```python
from build123d import *

# Parameters (mm, degrees)
SKETCH_1_R          = 16
SKETCH_1_R_2        = 1.2
EXTRUDE_1_DEPTH     = 3.6
SKETCH_2_R          = 2
CUT_EXTRUDE_1_DEPTH = 2
SKETCH_3_R          = 1
CUT_EXTRUDE_2_DEPTH = 2
SKETCH_4_R          = 7.9
EXTRUDE_2_DEPTH     = 10
SKETCH_6_R          = 0.7
CUT_EXTRUDE_3_DEPTH = 5


with BuildPart() as part:
    # 스케치1 → 보스-돌출1 (new body)
    with BuildSketch(Plane.XY):
        Circle(SKETCH_1_R)
        with Locations((13, 0)):
            Circle(SKETCH_1_R_2, mode=Mode.SUBTRACT)
        with Locations((6.5, -11.258330249)):
            Circle(SKETCH_1_R_2, mode=Mode.SUBTRACT)
        with Locations((-6.5, -11.258330249)):
            Circle(SKETCH_1_R_2, mode=Mode.SUBTRACT)
        with Locations((-13, 0)):
            Circle(SKETCH_1_R_2, mode=Mode.SUBTRACT)
        with Locations((-6.5, 11.258330249)):
            Circle(SKETCH_1_R_2, mode=Mode.SUBTRACT)
        with Locations((6.5, 11.258330249)):
            Circle(SKETCH_1_R_2, mode=Mode.SUBTRACT)
    extrude(amount=EXTRUDE_1_DEPTH)

    # 스케치2 → 컷-돌출1 (cut)
    with BuildSketch(Plane.XY.offset(3.6)):
        with Locations((13, 0)):
            Circle(SKETCH_2_R)
        with Locations((6.5, -11.258330249)):
            Circle(SKETCH_2_R)
        with Locations((-6.5, -11.258330249)):
            Circle(SKETCH_2_R)
        with Locations((-13, 0)):
            Circle(SKETCH_2_R)
        with Locations((-6.5, 11.258330249)):
            Circle(SKETCH_2_R)
        with Locations((6.5, 11.258330249)):
            Circle(SKETCH_2_R)
    extrude(amount=-CUT_EXTRUDE_1_DEPTH, mode=Mode.SUBTRACT)

    # 스케치3 → 컷-돌출2 (cut)
    with BuildSketch(Plane(origin=(0, 0, 0), x_dir=(-1, 0, 0), z_dir=(0, 0, -1))):
        with Locations((-6, 0)):
            Circle(SKETCH_3_R)
        with Locations((6, 0)):
            Circle(SKETCH_3_R)
    extrude(amount=-CUT_EXTRUDE_2_DEPTH, mode=Mode.SUBTRACT)

    # 스케치4 → 보스-돌출2 (add)
    with BuildSketch(Plane.XY.offset(3.6)):
        Circle(SKETCH_4_R)
    extrude(amount=EXTRUDE_2_DEPTH)

    # 스케치5 → 컷-회전1 (revolve, cut)
    with BuildSketch(Plane(origin=(0, 0, 0), x_dir=(0, 0, -1), z_dir=(1, 0, 0))):
        Polygon((-13.6, 7.9), (-13.6, 5.9), (-12.35, 4.6), (-11.1, 5.9), (-11.1, 7.9), align=None)
        Polygon((-6.1, 7.9), (-3.6, 7.9), (-3.6, 5.9), (-4.85, 4.6), (-6.1, 5.9), align=None)
    revolve(axis=Axis((0, 0, 0), (0, 0, 1)), mode=Mode.SUBTRACT)

    # 스케치6 → 컷-돌출3 (cut)
    with BuildSketch(Plane.XY.offset(11.1)):
        with Locations((6.6, 0)):
            Circle(SKETCH_6_R)
    extrude(amount=-CUT_EXTRUDE_3_DEPTH, mode=Mode.SUBTRACT)


solid = part.part
```
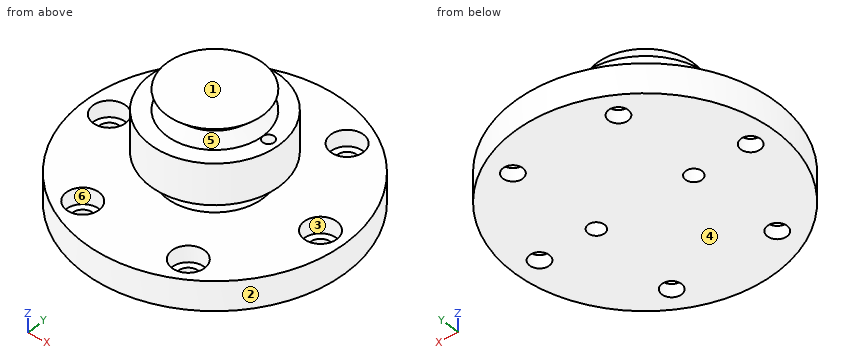
Input: part model. Units: mm. Frame: model coordinates. Face numbers are marked on the shaded views. A direction names the side the tool comes from. Give positions to 0.01 mm unless a question says otherwise; leave off trailing zeros. Order: outer loops, then holes, each group sorted by start corner. A loop starts at its lowest first (then second) coordinate and runs counter-clockwise, first axis right, second up. Notation, with made-up numbers: M 25,-39 L 31,-39 A20 cw 31,-12 Z; hole C -27,8.25 d2. An arc over 180 degrees is marked long. Return JSON: item names as keys, results as strings.
1) Section query C-C on x = -6.5. Output: boundary loops of the cut face in (y, z), and give its area (3 significant figures).
Taken from the geometry:
{"outline": "M -14.62,0 L -12.46,0 L -12.46,1.6 L -13.26,1.6 L -13.26,3.6 L -14.62,3.6 Z; M -10.06,0 L -0.87,0 L -0.87,2 L 0.87,2 L 0.87,0 L 10.06,0 L 10.06,1.6 L 9.26,1.6 L 9.26,3.6 L -9.26,3.6 L -9.26,1.6 L -10.06,1.6 Z; M -4.49,6.1 L 4.49,6.1 L 4.49,11.1 L -4.49,11.1 Z; M 12.46,0 L 14.62,0 L 14.62,3.6 L 13.26,3.6 L 13.26,1.6 L 12.46,1.6 Z", "area": "123 mm2"}
2) Section query D-D on x = 0. Output: boundary loops of the cut face in (y, z), and give its area (3 significant figures).
Taken from the geometry:
{"outline": "M -16,0 L 16,0 L 16,3.6 L 5.9,3.6 L 4.6,4.85 L 5.9,6.1 L 7.9,6.1 L 7.9,11.1 L 5.9,11.1 L 4.6,12.35 L 5.9,13.6 L -5.9,13.6 L -4.6,12.35 L -5.9,11.1 L -7.9,11.1 L -7.9,6.1 L -5.9,6.1 L -4.6,4.85 L -5.9,3.6 L -16,3.6 Z", "area": "247 mm2"}
3) Line query: L1, parallel to Y at x = 7, z = 2.5; L2, parallel to Y at x = -6.5, z = 0.5; L3, parallel to Y at x = 0, z = 7.5. Output: solid intervals per line, ascending. Write a range as [from, to].
Taken from the geometry:
{"L1": "y = [-14.39, -13.19], [-9.32, 9.32], [13.19, 14.39]", "L2": "y = [-14.62, -12.46], [-10.06, -0.87], [0.87, 10.06], [12.46, 14.62]", "L3": "y = [-7.9, 7.9]"}
4) Contact query for flat-ended pins moving along their axis: pin 1 (4 mm diameter, centred on x = 2, z = 12, fed in from +Y); pin 2 (1.5 mm diameter, centred on x = -2.5, z = 7.5, fed in from +Y); pin 3 (17.5 mm diameter, centred on x = 3.5, y = -1.5, fed in from -Z); pin 4 (6.5 mm diameter, centred on x = -6.5, y = -11.26, fed in from +Z). Output: stop coordinate, or through.
Taken from the geometry:
{"pin 1": "stops at y = 7.9", "pin 2": "stops at y = 7.7", "pin 3": "stops at z = 0", "pin 4": "stops at z = 3.6"}
5) Section query A-A on x = 6.6. Count the separate pieces of the cut face and the enclosed holes in it, and give its area (3 significant figures).
Taken from the geometry:
{"separate pieces": "5", "enclosed holes": "0", "area": "115 mm2"}
6) Mould query, pull axis X, two halves, no side actions, for the marked faces 1, 2 and 3. Classes: released by +X, released by -X, zero draft, split by the parting line, or undercut.
Taken from the geometry:
{"face 1": "zero draft", "face 2": "split by the parting line", "face 3": "undercut"}
7) Access query for the marked faces 4, 5 and 6. Directions: +Z, -Z, +X, -X, +Y, -Y. A direction counts if a zero-diameter tool reaches every point of the face in a straight line with its end or side. Return the directions, or none.
Taken from the geometry:
{"face 4": "-Z, +X, -X, +Y, -Y", "face 5": "none", "face 6": "+Z"}
8) Section query B-B on z = 10.25. Output: boundary loops of the cut face in (x, y), and give its area (3 significant figures).
Taken from the geometry:
{"outline": "C 0,0 d15.8; hole C 6.6,0 d1.4", "area": "195 mm2"}
